from build123d import *

# Parameters (mm, degrees)
F0_W     = 31
F0_H     = 13
F1_DEPTH = 0.7
F2_R     = 1.55
F3_DEPTH = 25
F4_R     = 2


with BuildPart() as f1:
    # F0 (on Front) → F1 (new body)
    with BuildSketch(Plane.XZ):
        with Locations((15.5, 6.5)):
            Rectangle(F0_W, F0_H)
    extrude(amount=F1_DEPTH)

    # F2 (on face) → F3 (cut)
    with BuildSketch(Plane.XZ.offset(0.7)):
        with Locations((4, 10)):
            Circle(F2_R)
        with Locations((4, 3)):
            Circle(F2_R)
        with Locations((27, 10)):
            Circle(F2_R)
        with Locations((27, 3)):
            Circle(F2_R)
    extrude(amount=-F3_DEPTH, mode=Mode.SUBTRACT)

    # F4
    f4_edges = [f1.edges().sort_by_distance(p)[0] for p in [
        (31, -0.35, 13),
        (31, -0.35, 0),
        (0, -0.35, 0),
        (0, -0.35, 13),
    ]]
    fillet(f4_edges, radius=F4_R)


solid = f1.part
The listing builds one solid part. Answer for the finished solid, in the listing's coordinates (mm). Give positions to 0.01 mm unless a question says otherwise; leave off trailing zeros. Write each loop counter-clockwise with the first axis right and the second up, starting at its lowest first coordinate (ties: lowest second). Pieces come first, ordered by that corner, then holes. Notation, with made-up numbers: (-22, 84.25) -> (11, 84.25) arc R25 cw to (11, 109.25) -> close; hole circle Ø8 at (64, 70.5). An arc over 180 degrees is marked (long way). One line per question, with ' | ' between items. Start each with the question number.
1. Given pin 1 Ø4 at (x, z) = (27, 3) entering from -Y, flat-ended and moving along its own axis, determine where the tip first touches the part or whether it passes through.
2. Section D-D (z = 1) is taken. Determine the outline of the cut face in (x, y).
3. Section A-A (z = 10) is taken. Determine the outline of the cut face in (x, y).
4. Section C-C (x = 27) is taken. Determine the outline of the cut face in (y, z).
5. Find the intervals of material crossed by probe 1 along Z at (x, y) = (4, -0.3); probe 2 along X at (y, z) = (-0.5, 2.25); probe 3 along Z at (x, y) = (3, -0.45), in increasing order.
6. For a pull along X with two mould halves and no side action, classify faces 1 (the cylindrical face through (2.45, -0.35, 10.07)), 2 (the cylindrical face through (0.57, -0.35, 12.4)), 3 (the cylindrical face through (30.4, -0.35, 12.43)) as pulls with the +X half, pulls with the -X half, needs draft (parallel to the pull), parting line crosses it, or undercut.
7. Section B-B (y = -0.5) is taken. Determine the outline of the cut face in (x, z).
Response values:
1) pin 1: y = -0.7
2) outline: (0.27, -0.7) -> (30.73, -0.7) -> (30.73, 0) -> (0.27, 0) -> close
3) outline: (0, -0.7) -> (2.45, -0.7) -> (2.45, 0) -> (0, 0) -> close; (5.55, -0.7) -> (25.45, -0.7) -> (25.45, 0) -> (5.55, 0) -> close; (28.55, -0.7) -> (31, -0.7) -> (31, 0) -> (28.55, 0) -> close
4) outline: (-0.7, 0) -> (0, 0) -> (0, 1.45) -> (-0.7, 1.45) -> close; (-0.7, 4.55) -> (0, 4.55) -> (0, 8.45) -> (-0.7, 8.45) -> close; (-0.7, 11.55) -> (0, 11.55) -> (0, 13) -> (-0.7, 13) -> close
5) probe 1: 0 to 1.45, 4.55 to 8.45, 11.55 to 13 | probe 2: 0 to 2.64, 5.36 to 25.64, 28.36 to 31 | probe 3: 0 to 1.82, 4.18 to 8.82, 11.18 to 13
6) face 1: undercut | face 2: pulls with the -X half | face 3: pulls with the +X half
7) outline: (0, 2) arc R2 ccw to (2, 0) -> (29, 0) arc R2 ccw to (31, 2) -> (31, 11) arc R2 ccw to (29, 13) -> (2, 13) arc R2 ccw to (0, 11) -> close; hole circle Ø3.1 at (4, 3); hole circle Ø3.1 at (4, 10); hole circle Ø3.1 at (27, 3); hole circle Ø3.1 at (27, 10)
